Input: dimensioned drawing with shaded views. Units: mm. Origin: part minimum x, y, z. Give positions to 0.01 mm unless a question says otherwise; leave off trailing zeros. Write each loop counter-clockwise with the first axis right and the second up, starting at its lowest first coordinate (ties: lowest second). Pieces come first, ordered by that corner, then holes. Notation, with made-up numbers: (79, 41.25) -> (101, 41.25) arc R16 ccw to (101, 60.25) -> close; hole circle Ø5 at (-11, 68.5). An arc over 180 degrees is marked (long way). Return JSON: item names as keys, results as strings. Group by question number.
Item 1: Line query: line 1 (Z direction, x = 27, y = 11); line 2 (X direction, y = 8.25, z = 18.5); line 3 (X direction, y = 12, z = 27). Output: solid intervals per line, ascending. Write a range as [from, to].
Item 2: Section A-A, the plane y = 11. Return loops of the section in (x, z), then the cut area to 3 significant figures.
Item 3: Section C-C, the plane z = 15. Return loops of the section in (x, y).
Item 4: Section D-D, the plane z = 20. Return loops of the section in (x, y), then the cut area to 3 significant figures.
Item 5: Pin query (flat end, axial travel): P1, Ø4, axis at y = 7, z = 14, coming from the -X side; P2, Ø8, axis at x = 24, z = 23, coming from the -Y side; P3, Ø1, axis at y = 3, z = 20, coming from the -X side. Return the tip coordinate at first contact, or that it passes through.
Item 6: Section B-B, the plane x = 13. Return loops of the section in (y, z).
Item 7: Mould query, pull axis Y, two halves, no side actions, for the marked faces 1, 2 and 3. Classes: released by +Y, released by -Y, zero draft, split by the parting line, or undercut.
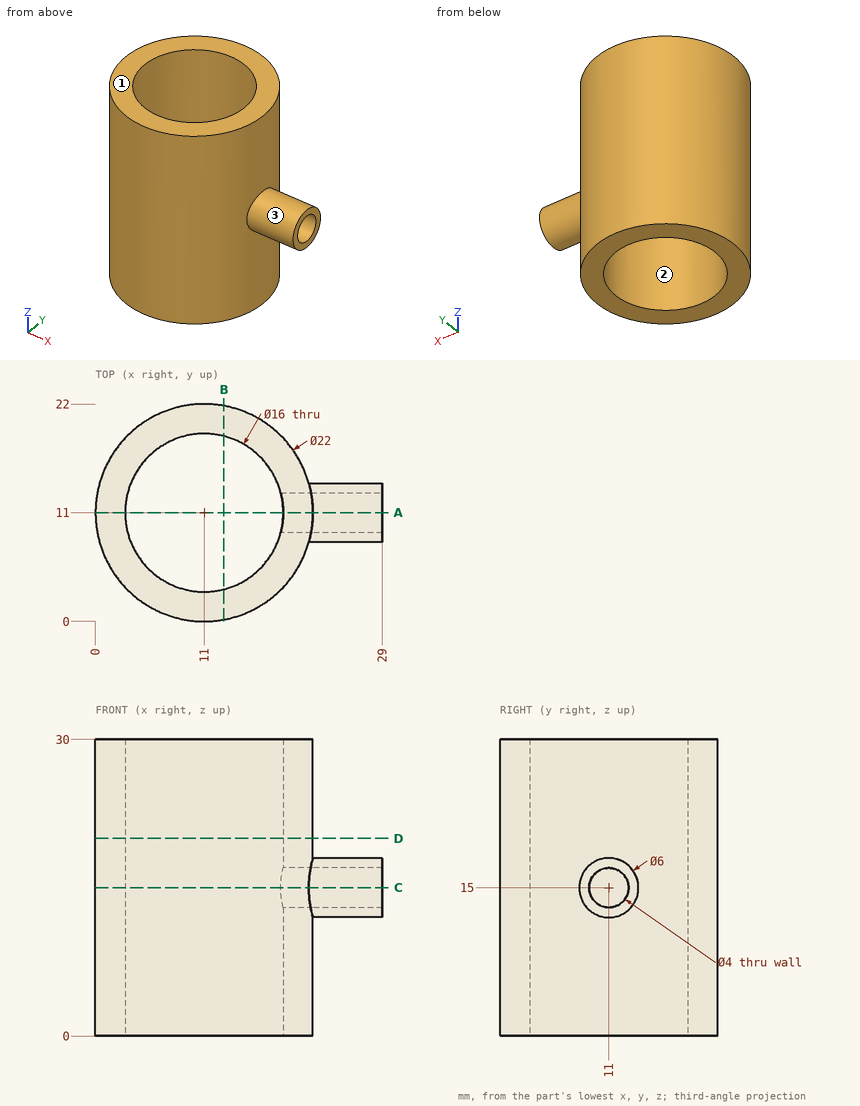
Answer below:
{
 "1": {"line 1": "z = [12, 13], [17, 18]", "line 2": "x = [0.35, 3.49], [18.51, 21.65]", "line 3": "x = [0.05, 3.06], [18.94, 21.95]"},
 "2": {"outline": "(0, 0) -> (3, 0) -> (3, 30) -> (0, 30) -> close; (19, 0) -> (22, 0) -> (22, 12) -> (29, 12) -> (29, 13) -> (19, 13) -> close; (19, 17) -> (29, 17) -> (29, 18) -> (22, 18) -> (22, 30) -> (19, 30) -> close", "area": "182 mm2"},
 "3": {"outline": "(18.75, 9) arc R8 cw (long way) to (18.75, 13) -> (29, 13) -> (29, 14) -> (21.58, 14) arc R11 ccw (long way) to (21.58, 8) -> (29, 8) -> (29, 9) -> close"},
 "4": {"outline": "circle Ø22 at (11, 11); hole circle Ø16 at (11, 11)", "area": "179 mm2"},
 "5": {"P1": "stops at x = 0.18", "P2": "stops at y = 4.68", "P3": "stops at x = 2.95"},
 "6": {"outline": "(0.18, 0) -> (3.25, 0) -> (3.25, 30) -> (0.18, 30) -> close; (18.75, 0) -> (21.82, 0) -> (21.82, 30) -> (18.75, 30) -> close"},
 "7": {"face 1": "zero draft", "face 2": "undercut", "face 3": "split by the parting line"}
}
